from build123d import *

# Parameters (mm, degrees)
F1_DEPTH = 8
F2_DEPTH = 8
F3_DEPTH = 4


with BuildPart() as f1:
    # F0 (on Top) → F1 (new body)
    with BuildSketch(Plane.XY):
        with BuildLine():
            Line((31.5, 26.5), (-31.5, 26.5))
            ThreePointArc((-31.5, 26.5), (-35.0355339059, 25.0355339059), (-36.5, 21.5))
            Line((-36.5, 21.5), (-36.5, -21.5))
            ThreePointArc((-36.5, -21.5), (-35.0355339059, -25.0355339059), (-31.5, -26.5))
            Line((-31.5, -26.5), (31.5, -26.5))
            ThreePointArc((31.5, -26.5), (35.0355339059, -25.0355339059), (36.5, -21.5))
            Line((36.5, -21.5), (36.5, 21.5))
            ThreePointArc((36.5, 21.5), (35.0355339059, 25.0355339059), (31.5, 26.5))
        make_face()
        with BuildLine():
            ThreePointArc((-34.5, 19.5), (-33.0355339059, 23.0355339059), (-29.5, 24.5))
            Line((-29.5, 24.5), (29.5, 24.5))
            ThreePointArc((29.5, 24.5), (33.0355339059, 23.0355339059), (34.5, 19.5))
            Line((34.5, 19.5), (34.5, -19.5))
            ThreePointArc((34.5, -19.5), (33.0355339059, -23.0355339059), (29.5, -24.5))
            Line((29.5, -24.5), (-29.5, -24.5))
            ThreePointArc((-29.5, -24.5), (-33.0355339059, -23.0355339059), (-34.5, -19.5))
            Line((-34.5, -19.5), (-34.5, 19.5))
        make_face(mode=Mode.SUBTRACT)
        with BuildLine():
            Line((29.5, 24.5), (-29.5, 24.5))
            ThreePointArc((-29.5, 24.5), (-33.0355339059, 23.0355339059), (-34.5, 19.5))
            Line((-34.5, 19.5), (-34.5, -19.5))
            ThreePointArc((-34.5, -19.5), (-33.0355339059, -23.0355339059), (-29.5, -24.5))
            Line((-29.5, -24.5), (29.5, -24.5))
            ThreePointArc((29.5, -24.5), (33.0355339059, -23.0355339059), (34.5, -19.5))
            Line((34.5, -19.5), (34.5, 19.5))
            ThreePointArc((34.5, 19.5), (33.0355339059, 23.0355339059), (29.5, 24.5))
        make_face()
    extrude(amount=F1_DEPTH)

    # F0 (on Top) → F2 (join)
    with BuildSketch(Plane.XY):
        with BuildLine():
            Line((31.5, 26.5), (-31.5, 26.5))
            ThreePointArc((-31.5, 26.5), (-35.0355339059, 25.0355339059), (-36.5, 21.5))
            Line((-36.5, 21.5), (-36.5, -21.5))
            ThreePointArc((-36.5, -21.5), (-35.0355339059, -25.0355339059), (-31.5, -26.5))
            Line((-31.5, -26.5), (31.5, -26.5))
            ThreePointArc((31.5, -26.5), (35.0355339059, -25.0355339059), (36.5, -21.5))
            Line((36.5, -21.5), (36.5, 21.5))
            ThreePointArc((36.5, 21.5), (35.0355339059, 25.0355339059), (31.5, 26.5))
        make_face()
        with BuildLine():
            ThreePointArc((-34.5, 19.5), (-33.0355339059, 23.0355339059), (-29.5, 24.5))
            Line((-29.5, 24.5), (29.5, 24.5))
            ThreePointArc((29.5, 24.5), (33.0355339059, 23.0355339059), (34.5, 19.5))
            Line((34.5, 19.5), (34.5, -19.5))
            ThreePointArc((34.5, -19.5), (33.0355339059, -23.0355339059), (29.5, -24.5))
            Line((29.5, -24.5), (-29.5, -24.5))
            ThreePointArc((-29.5, -24.5), (-33.0355339059, -23.0355339059), (-34.5, -19.5))
            Line((-34.5, -19.5), (-34.5, 19.5))
        make_face(mode=Mode.SUBTRACT)
    extrude(amount=F2_DEPTH)

    # F0 (on Top) → F3 (cut)
    with BuildSketch(Plane.XY):
        with BuildLine():
            Line((31.5, 26.5), (-31.5, 26.5))
            ThreePointArc((-31.5, 26.5), (-35.0355339059, 25.0355339059), (-36.5, 21.5))
            Line((-36.5, 21.5), (-36.5, -21.5))
            ThreePointArc((-36.5, -21.5), (-35.0355339059, -25.0355339059), (-31.5, -26.5))
            Line((-31.5, -26.5), (31.5, -26.5))
            ThreePointArc((31.5, -26.5), (35.0355339059, -25.0355339059), (36.5, -21.5))
            Line((36.5, -21.5), (36.5, 21.5))
            ThreePointArc((36.5, 21.5), (35.0355339059, 25.0355339059), (31.5, 26.5))
        make_face()
        with BuildLine():
            ThreePointArc((-34.5, 19.5), (-33.0355339059, 23.0355339059), (-29.5, 24.5))
            Line((-29.5, 24.5), (29.5, 24.5))
            ThreePointArc((29.5, 24.5), (33.0355339059, 23.0355339059), (34.5, 19.5))
            Line((34.5, 19.5), (34.5, -19.5))
            ThreePointArc((34.5, -19.5), (33.0355339059, -23.0355339059), (29.5, -24.5))
            Line((29.5, -24.5), (-29.5, -24.5))
            ThreePointArc((-29.5, -24.5), (-33.0355339059, -23.0355339059), (-34.5, -19.5))
            Line((-34.5, -19.5), (-34.5, 19.5))
        make_face(mode=Mode.SUBTRACT)
    extrude(amount=F3_DEPTH, mode=Mode.SUBTRACT)


solid = f1.part
Design review of the part built by this model. Coordinates are the model's own, in mm. A direction names the side the tool comes from. Coordinates: 2 decimals unless noted, no trailing zeros. Order: outer loops, then holes, each group sorted by start corner. A loop starts at its lowest first (then second) coordinate and runs counter-clockwise, first axis right, second up. Notation, with made-up numbers: (40.5, -27) - (80.5, -27) arc R15 ccw to (80.5, -22) - close; hole circle Ø11 at (-40, 21). An arc over 180 degrees is marked (long way). Put each result on its own line as item: value.
1) Tool access review of faces 1 (the face through (-34.5, 0, 2)), 2 (the face through (0, 26, 4)), 3 (the face through (33.07, -23, 1.97)), 4 (the face through (33, 23.07, 1.97)), 5 (the face through (-33.07, 23, 1.97)): name each direction out of +Z, -Z, +X, -X, +Y, -Y from which nothing blocks a thin tool from reaching the whole face with its end or side.
Response values:
face 1: -Z, -X, +Y, -Y
face 2: -Z
face 3: -Z, +X, -Y
face 4: -Z, +X, +Y
face 5: -Z, -X, +Y
2) Wall thickness on L1, parallel to X at y = -5, z = 1.75; L2, parallel to Y at x = 13, z = 1.5; L3, parallel to X at y = -23, z = 2.25: over which ranges is each line inside the solid? List them lowest first. Write a range as from..to.
Response values:
L1: x = -34.5..34.5
L2: y = -24.5..24.5
L3: x = -33.07..33.07
3) Take a section at A-A, the plane z = 2.25. Give the boundary of the cut face in (x, y).
Response values:
outline: (-34.5, -19.5) arc R5 ccw to (-29.5, -24.5) - (29.5, -24.5) arc R5 ccw to (34.5, -19.5) - (34.5, 19.5) arc R5 ccw to (29.5, 24.5) - (-29.5, 24.5) arc R5 ccw to (-34.5, 19.5) - close
4) Take a section at B-B, the plane x = 17. Give the boundary of the cut face in (y, z).
Response values:
outline: (-26.5, 4) - (-24.5, 4) - (-24.5, 0) - (24.5, 0) - (24.5, 4) - (26.5, 4) - (26.5, 8) - (-26.5, 8) - close
5) Insertion check: P1, Ø4.5, axis at x = 0.5, z = 1.5, coming from the -Y side; P2, Ø3, axis at y = 2, z = 1, coming from the -X side; P3, Ø3, axis at x = 9, z = 2, coming from the +Y side. Each pin has a flat end and moves straight along its axis. Give the tip position at first contact, or say it passes through.
Response values:
P1: stops at y = -24.5
P2: stops at x = -34.5
P3: stops at y = 24.5
